The listing builds one solid part. Answer for the finished solid, in the listing's coordinates (mm). A direction names the side the tool comes from. Give positions to 0.01 mm unless a question says otherwise; leave off trailing zeros. Order: outer loops, then holes, each group sorted by start corner. A loop starts at its lowest first (then second) coordinate and runs counter-clockwise, first axis right, second up. Notation, with made-up numbers: (-2, 61) - (21, 61) arc R28 cw to (21, 82) - close; hole circle Ø1 at (82, 66.25). An arc over 180 degrees is marked (long way). Answer as a JSON object with one key per item and string values. Group by question number.
Q1. A cutting plane is placed at C-C, the plane y = 28. Give the vertices of the cut face in (x, z), and give its area (3 significant figures).
Q2. A cutting plane is placed at B-B, the plane z = 4.25. Count the separate pieces of the cut face and the enclosed holes in it, and give its area (3 significant figures).
Q3. Consider line 1 (X direction, y = -23.5, z = 1.5); line 2 (X direction, y = 4, z = 4); line 3 (X direction, y = -32.5, z = 3.25). Determine where each line is inside the solid, lowest interval first.
Q4. A cutting plane is placed at A-A, the plane x = -17. Give the vertices of the cut face in (y, z), and give its area (3 significant figures).
Q5. The mould has two halves that part along Y. Classify faces 5 (the face through (-14.759, 1.004, 3.131)), 6 (the face through (14.44, 10.45, 3.13)), 7 (the face through (2.155, -19, 3)), 8 (the face through (-7.651, -34.055, 3.131)): released by +Y, released by -Y, zero draft, split by the parting line, or undercut.
Q6. For faces 1 (the face through (14, -6.589, 3)), 2 (the face through (17, -11.658, 3)), 3 (the face through (24.144, 22.148, 3.131)), 4 (the face through (-1.036, -2, 3)), determine the directions among +Z, -Z, +X, -X, +Y, -Y from which every point of the face is accessible in a straight line to the end or side of a thin tool.
Q7. Given pin 1 (2.5 mm diameter, centred on x = 7.5, z = 2, fed in from +Y); pin 2 (1.2 mm diameter, centred on y = 11, z = 4, fed in from +X); pin 3 (1.3 mm diameter, centred on x = -19, z = 1.5, fed in from +Y); pin 4 (12 mm diameter, centred on x = 18.5, y = -19, fed in from -Z), each flat-ended and moving along its own axis, determine where each tip first touches the part or whether it passes through.
from build123d import *

# Parameters (mm, degrees)
F1_DEPTH = 6.35


with BuildPart() as f1:
    # F0 (on Top) → F1 (new body)
    with BuildSketch(Plane.XY):
        with BuildLine():
            ThreePointArc((23.402542, 23.817074), (-3.062865, 38.874712), (-29.25491, 23.346445))
            Line((-29.25491, 23.346445), (-30.065471, 17.915688))
            Line((-30.065471, 17.915688), (-30.065471, 15.159781))
            Line((-30.065471, 15.159781), (-30.065471, 12.403875))
            Line((-30.065471, 12.403875), (-30.065471, 9.891136))
            Line((-30.065471, 9.891136), (-29.417021, 5.838332))
            Line((-29.417021, 5.838332), (-28.282236, 2.515032))
            Line((-28.282236, 2.515032), (-26.417948, 0))
            Line((-26.417948, 0), (-24.796825, -1.861996))
            Line((-24.796825, -1.861996), (-25.589179, -2.551849))
            Line((-25.589179, -2.551849), (-26.808415, -3.101752))
            ThreePointArc((-26.808415, -3.101752), (-27.185988, -7.708848), (-24.735437, -11.628375))
            Line((-24.735437, -11.628375), (-22.263491, -10.76789))
            Line((-22.263491, -10.76789), (-19.924534, -11.628375))
            Line((-19.924534, -11.628375), (-18.360017, -11.628375))
            Line((-18.360017, -11.628375), (-17.880529, -10.806396))
            Line((-17.880529, -10.806396), (-18.360017, -10.526695))
            Line((-18.360017, -10.526695), (-19.924534, -10.526695))
            Line((-19.924534, -10.526695), (-19.142276, -9.046921))
            Line((-19.142276, -9.046921), (-15.700337, -7.091273))
            Line((-15.700337, -7.091273), (-14.057593, -6.38724))
            Line((-14.057593, -6.38724), (-12.5713, -6.38724))
            Line((-12.5713, -6.38724), (-12.336623, -7.267281))
            Line((-12.336623, -7.267281), (-12.336623, -11.628375))
            Line((-12.336623, -11.628375), (-11.163235, -17.93534))
            Line((-11.163235, -17.93534), (-11.163235, -18.981609))
            Line((-11.163235, -18.981609), (-11.006783, -22.580002))
            Line((-11.006783, -22.580002), (-11.006783, -24.692101))
            Line((-11.006783, -24.692101), (-11.006783, -28.948328))
            Line((-11.006783, -28.948328), (-10.449933, -33.126414))
            Line((-10.449933, -33.126414), (-9.883413, -34.330271))
            Line((-9.883413, -34.330271), (-8.097164, -35.095806))
            Line((-8.097164, -35.095806), (-7.192442, -32.984786))
            Line((-7.192442, -32.984786), (-7.192442, -30.364629))
            Line((-7.192442, -30.364629), (-7.192442, -26.682248))
            Line((-7.192442, -26.682248), (-7.192442, -22.999866))
            Line((-7.192442, -22.999866), (-7.192442, -19.388299))
            Line((-7.192442, -19.388299), (-7.192442, -13.439838))
            Line((-7.192442, -13.439838), (-6.413477, -16.838958))
            Line((-6.413477, -16.838958), (-6.413477, -20.521341))
            Line((-6.413477, -20.521341), (-6.413477, -24.557797))
            Line((-6.413477, -24.557797), (-6.413477, -28.806698))
            Line((-6.413477, -28.806698), (-6.413477, -34.542717))
            Line((-6.413477, -34.542717), (-6.413477, -35.959017))
            Line((-6.413477, -35.959017), (-2.872725, -35.959017))
            Line((-2.872725, -35.959017), (-2.872725, -15.210214))
            Line((-2.872725, -15.210214), (-2.022945, -13.227393))
            Line((-2.022945, -13.227393), (-1.456425, -14.431247))
            Line((-1.456425, -14.431247), (-1.456425, -16.484883))
            Line((-1.456425, -16.484883), (-1.456425, -21.158677))
            Line((-1.456425, -21.158677), (-1.456425, -36.029831))
            Line((-1.456425, -36.029831), (0, -36.029831))
            Line((0, -36.029831), (1.022101, -35.109237))
            Line((1.022101, -35.109237), (1.531237, -33.921254))
            Line((1.531237, -33.921254), (1.531237, -31.285223))
            Line((1.531237, -31.285223), (2.155141, -25.620023))
            Line((2.155141, -25.620023), (2.155141, -20.662971))
            Line((2.155141, -20.662971), (2.155141, -16.484883))
            Line((2.155141, -16.484883), (2.155141, -13.014947))
            Line((2.155141, -13.014947), (2.587357, -12.006444))
            Line((2.587357, -12.006444), (4.159939, -12.680407))
            Line((4.159939, -12.680407), (3.753364, -13.629085))
            Line((3.753364, -13.629085), (3.075737, -15.210214))
            Line((3.075737, -15.210214), (3.075737, -17.26385))
            Line((3.075737, -17.26385), (3.075737, -35.959017))
            Line((3.075737, -35.959017), (4.775298, -35.250865))
            Line((4.775298, -35.250865), (5.908338, -34.471899))
            Line((5.908338, -34.471899), (6.616489, -32.701526))
            Line((6.616489, -32.701526), (6.869, -30.408662))
            Line((6.869, -30.408662), (7.103555, -28.278847))
            Line((7.103555, -28.278847), (7.290181, -26.584241))
            Line((7.290181, -26.584241), (7.290181, -24.203721))
            Line((7.290181, -24.203721), (7.290181, -21.866826))
            Line((7.290181, -21.866826), (7.290181, -19.600745))
            Line((7.290181, -19.600745), (7.457498, -18.081469))
            Line((7.457498, -18.081469), (7.544803, -17.288722))
            Line((7.544803, -17.288722), (8.316048, -15.210214))
            Line((8.316048, -15.210214), (9.095014, -13.014947))
            Line((9.095014, -13.014947), (9.394606, -10.294581))
            Line((9.394606, -10.294581), (9.895026, -8.41949))
            Line((9.895026, -8.41949), (10.646053, -7.339889))
            Line((10.646053, -7.339889), (12.382803, -6.588862))
            Line((12.382803, -6.588862), (14.682825, -6.588862))
            Line((14.682825, -6.588862), (15.903244, -7.480707))
            Line((15.903244, -7.480707), (16.231818, -8.372552))
            Line((16.231818, -8.372552), (16.231818, -9.358275))
            Line((16.231818, -9.358275), (15.809365, -10.672572))
            Line((15.809365, -10.672572), (16.278757, -11.658295))
            Line((16.278757, -11.658295), (17.076723, -11.658295))
            Line((17.076723, -11.658295), (17.827751, -11.658295))
            Line((17.827751, -11.658295), (19.611441, -10.672572))
            Line((19.611441, -10.672572), (21.160433, -9.170517))
            Line((21.160433, -9.170517), (22.427792, -7.433767))
            Line((22.427792, -7.433767), (23.038002, -5.931713))
            Line((23.038002, -5.931713), (22.427792, -4.007206))
            Line((22.427792, -4.007206), (22.427792, -1.660245))
            Line((22.427792, -1.660245), (22.944123, 0.827532))
            Line((22.944123, 0.827532), (23.648212, 3.972458))
            Line((23.648212, 3.972458), (24.117604, 5.990844))
            Line((24.117604, 5.990844), (25.523951, 11.89182))
            Line((25.523951, 11.89182), (25.523951, 13.210032))
            Line((25.523951, 13.210032), (25.74341, 16.501874))
            Line((25.74341, 16.501874), (24.865583, 20.525234))
            Line((24.865583, 20.525234), (23.402542, 23.817074))
        make_face()
        Polygon((-3.250899, -3.01964), (-5.046938, -6.791321), (-5.944957, -4.875546), (-5.944957, -4.157131), (-4.388391, -2.061753), (-4.388391, -1.043998), (-2.831824, 0), (-2.831824, -0.98413), align=None, mode=Mode.SUBTRACT)
        Polygon((-1.035786, -1.402149), (-0.969216, -0.468996), (1.295493, -3.957871), (1.907576, -5.426871), (0.68341, -7.140704), (-1.035786, -3.558452), align=None, mode=Mode.SUBTRACT)
        Polygon((-24.221089, 12.671578), (-5.1312, 2.728927), (-8.855303, 1.25334), (-11.244349, 0.761477), (-13.633396, 0.761477), (-15.917044, 1.25334), (-20.484339, 2.518129), (-22.486921, 3.080258), (-23.084182, 3.57212), (-24.454372, 5.926034), (-25.262432, 8.244814), (-25.71916, 10.563594), (-25.71916, 12.109448), (-25.262432, 12.671578), align=None, mode=Mode.SUBTRACT)
        Polygon((3.62141, 1.55088), (0.867034, 2.65263), (6.681826, 5.774255), (9.803452, 7.671713), (13.108702, 9.752797), (15.801869, 11.160589), (18.801078, 12.323546), (20.453703, 12.323546), (21.249412, 11.772673), (21.249412, 9.936422), (20.514911, 6.69238), (18.801078, 3.570755), (16.413951, 2.346588), (12.312994, 1.428463), (8.640493, 0.816379), (6.314577, 0.816379), align=None, mode=Mode.SUBTRACT)
    extrude(amount=F1_DEPTH)


solid = f1.part
Reply:
{
 "1": {"outline": "(-26.05, 0) - (20.47, 0) - (20.47, 6.35) - (-26.05, 6.35) - close", "area": "295 mm^2"},
 "2": {"separate pieces": "1", "enclosed holes": "4", "area": "2,450 mm^2"},
 "3": {"line 1": "x = -11.01 to -7.19, -6.41 to -2.87, -1.46 to 2.16, 3.08 to 7.29", "line 2": "x = -28.79 to -23.33, -7.57 to 3.38, 19.04 to 23.65", "line 3": "x = -10.53 to -7.19, -6.41 to -2.87, -1.46 to 1.53, 3.08 to 6.64"},
 "4": {"outline": "(-7.83, 0) - (1.55, 0) - (1.55, 6.35) - (-7.83, 6.35) - close; (8.91, 0) - (35.34, 0) - (35.34, 6.35) - (8.91, 6.35) - close", "area": "227 mm^2"},
 "5": {"face 5": "undercut", "face 6": "undercut", "face 7": "zero draft", "face 8": "released by -Y"},
 "6": {"face 1": "+Z, -Z, -Y", "face 2": "+Z, -Z, +X, -Y", "face 3": "+Z, -Z, +X, +Y", "face 4": "+Z, -Z"},
 "7": {"pin 1": "stops at y = 37.5", "pin 2": "stops at x = 25.45", "pin 3": "stops at y = 34.58", "pin 4": "passes through"}
}
